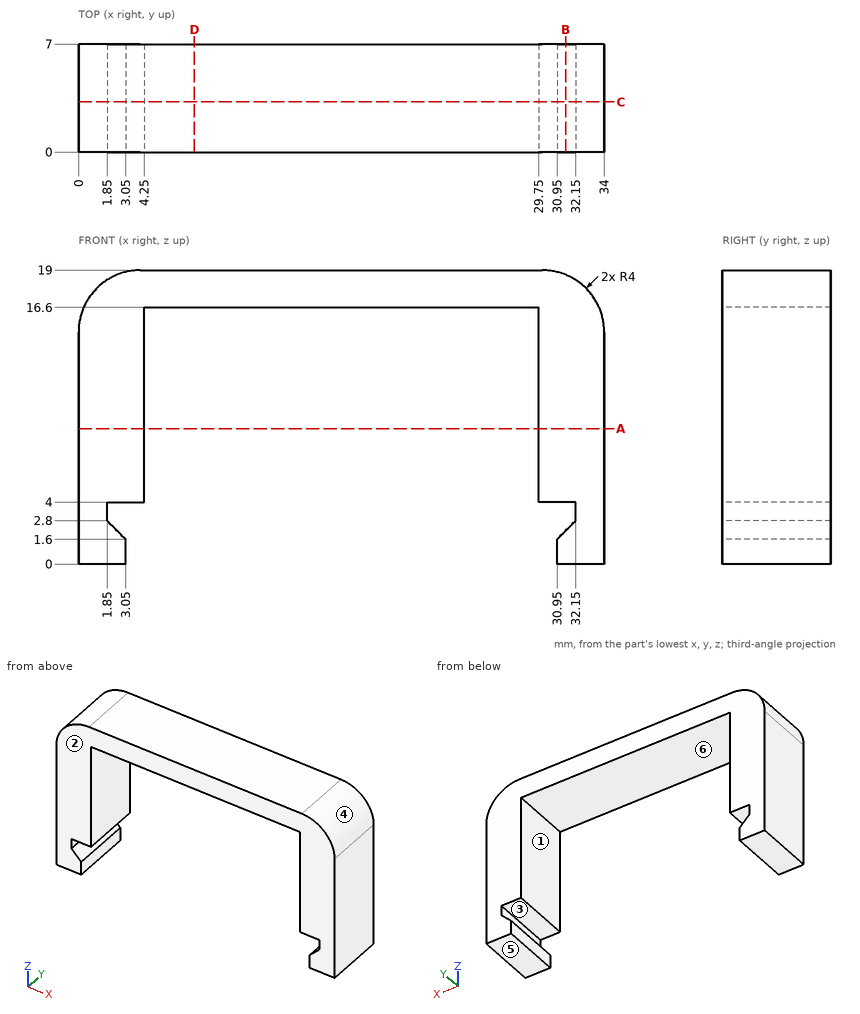
Study the drawing (mm; zero at the part's minimum x, y, z) and answer. A direction names the side the tool comes from. Round coordinates to 2 decimals unless told otherwise and drop trailing zeros. Write each loop counter-clockwise with the first axis right and the second up, starting at its lowest first coordinate (ties: lowest second). Pieces come first, ordered by that corner, then holes.
Q1. Straight lines are drawn through the part: line 1 (X direction, y = 4.5, z = 14.75); line 2 (Z direction, x = 25, y = 2); line 3 (Z direction, x = 3, y = 4.5). For each, find the intervals that lie inside material, in ascending order.
Values:
line 1: x = 0 to 4.25, 29.75 to 34
line 2: z = 16.6 to 19
line 3: z = 0 to 1.65, 4 to 18.87
Q2. A tool of negligible diameter and unlimited length cuts with its end or side. For the marked faces 1, 2 and 3, from which of +Z, -Z, +X, -X, +Y, -Y can it reach the whole face along a straight path? Write none if from no direction.
Values:
face 1: -Z, +Y, -Y
face 2: +Z, -Z, +X, -X, -Y
face 3: +Y, -Y
Q3. Find section B-B on x = 31.5. Determine the outline of the cut face in (y, z), and give its area (3 significant figures).
Values:
outline: (0, 0) - (7, 0) - (7, 2.15) - (0, 2.15) - close; (0, 4) - (7, 4) - (7, 18.71) - (0, 18.71) - close
area: 118 mm2
Q4. Find section A-A on z = 8.75. Determine the outline of the cut face in (x, y).
Values:
outline: (0, 0) - (4.25, 0) - (4.25, 7) - (0, 7) - close; (29.75, 0) - (34, 0) - (34, 7) - (29.75, 7) - close
Q5. Find section D-D on x = 7.5. Determine the outline of the cut face in (y, z), and give its area (3 significant figures).
Values:
outline: (0, 16.6) - (7, 16.6) - (7, 19) - (0, 19) - close
area: 16.8 mm2
Q6. The mould has two halves that part along X. Classify the marked faces 4, 5 and 6: released by +X, released by -X, zero draft, split by the parting line, or undercut.
Values:
face 4: released by +X
face 5: zero draft
face 6: undercut
Q7. Find section C-C on y = 3.25. Determine the outline of the cut face in (x, z).
Values:
outline: (0, 0) - (3.05, 0) - (3.05, 1.6) - (1.85, 2.8) - (1.85, 4) - (4.25, 4) - (4.25, 16.6) - (29.75, 16.6) - (29.75, 4) - (32.15, 4) - (32.15, 2.8) - (30.95, 1.6) - (30.95, 0) - (34, 0) - (34, 15) arc R4 ccw to (30, 19) - (4, 19) arc R4 ccw to (0, 15) - close
